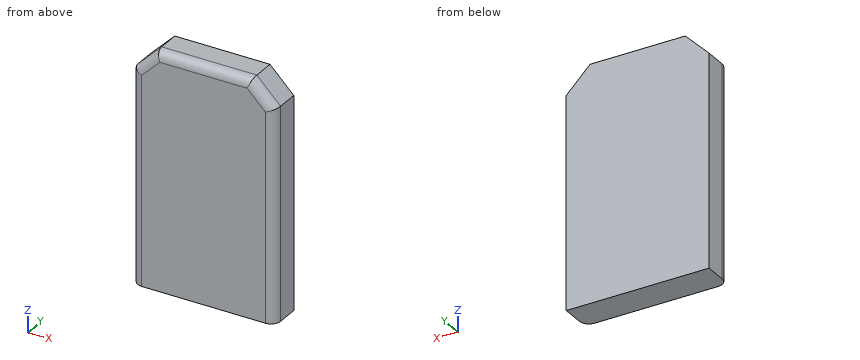
```python
from build123d import *

# Parameters (mm, degrees)
F0_W     = 30.0269816071
F0_H     = 49.5728440583
F1_DEPTH = 6.6
F2_SIZE  = 5
F3_R     = 2


with BuildPart() as f1:
    # F0 (on Front) → F1 (new body)
    with BuildSketch(Plane.XZ):
        Rectangle(F0_W, F0_H)
    extrude(amount=F1_DEPTH)

    # F2
    f2_edges = [f1.edges().sort_by_distance(p)[0] for p in [
        (-15.013491, -3.3, 24.786422),
        (15.013491, -3.3, 24.786422),
    ]]
    chamfer(f2_edges, length=F2_SIZE)

    # F3
    f3_edges = [f1.edges().sort_by_distance(p)[0] for p in [
        (12.513491, -6.6, 22.286422),
        (-15.013491, -6.6, -2.5),
        (0, -6.6, 24.786422),
        (15.013491, -6.6, -2.5),
        (-12.513491, -6.6, 22.286422),
    ]]
    fillet(f3_edges, radius=F3_R)


solid = f1.part
```
Model file for the job. Use its own axes, mm. Round coordinates to 2 decimals unless told otherwise and drop trailing zeros. Write each loop counter-clockwise with the first axis right and the second up, starting at its lowest first coordinate (ties: lowest second). Pieces come first, ordered by that corner, then holes. Notation, with made-up numbers: (42.5, 55.5) - (91.5, 55.5) arc R21 cw to (91.5, 90.5) - close; hole circle Ø3 at (33.5, 26). An arc over 180 degrees is marked (long way). Use CSV: the item, a comma, the result in double quotes. Start each with the question number.
Item 1: Drill centre lines: L1, parallel to Y at x = 13.5, z = -9; L2, parallel to Z at x = -13, y = -2.25; L3, parallel to Z at x = 13.5, y = -4.75. Where is each one in solid material? Low to high. Write a range as [from, to].
Item 2: Band-saw the part on A-A (y = -2.25). Write the cut outline in (x, z), and give its area (3 significant figures).
Item 3: Pin check, flat tip, straight feed: P1, Ø5, axis at x = 7.5, z = -5, coming from the +Y side. Stop position of the tip, or through.
Checked values:
1,L1,"y = [-6.54, 0]"
1,L2,"z = [-24.79, 21.8]"
1,L3,"z = [-24.79, 21.29]"
2,outline,"(-15.01, -24.79) - (15.01, -24.79) - (15.01, 19.79) - (10.01, 24.79) - (-10.01, 24.79) - (-15.01, 19.79) - close"
2,area,"1,460 mm²"
3,P1,"stops at y = 0"
